Drawing for the job (mm, zero at the part's lowest x, y, z). Round coordinates to 2 decimals unless told otherwise and drop trailing zeros. Write each loop counter-clockwise with the first axis right and the second up, starting at its lowest first coordinate (ties: lowest second). Pieces come first, ordered by that corner, then holes. Notation, with made-up numbers: (4.25, -35) - (46.25, -35) arc R26 ccw to (46.25, -15) - close; hole circle Ø9 at (26, 72.25). An arc over 180 degrees is marked (long way). Answer in a Markdown table with one row per item.
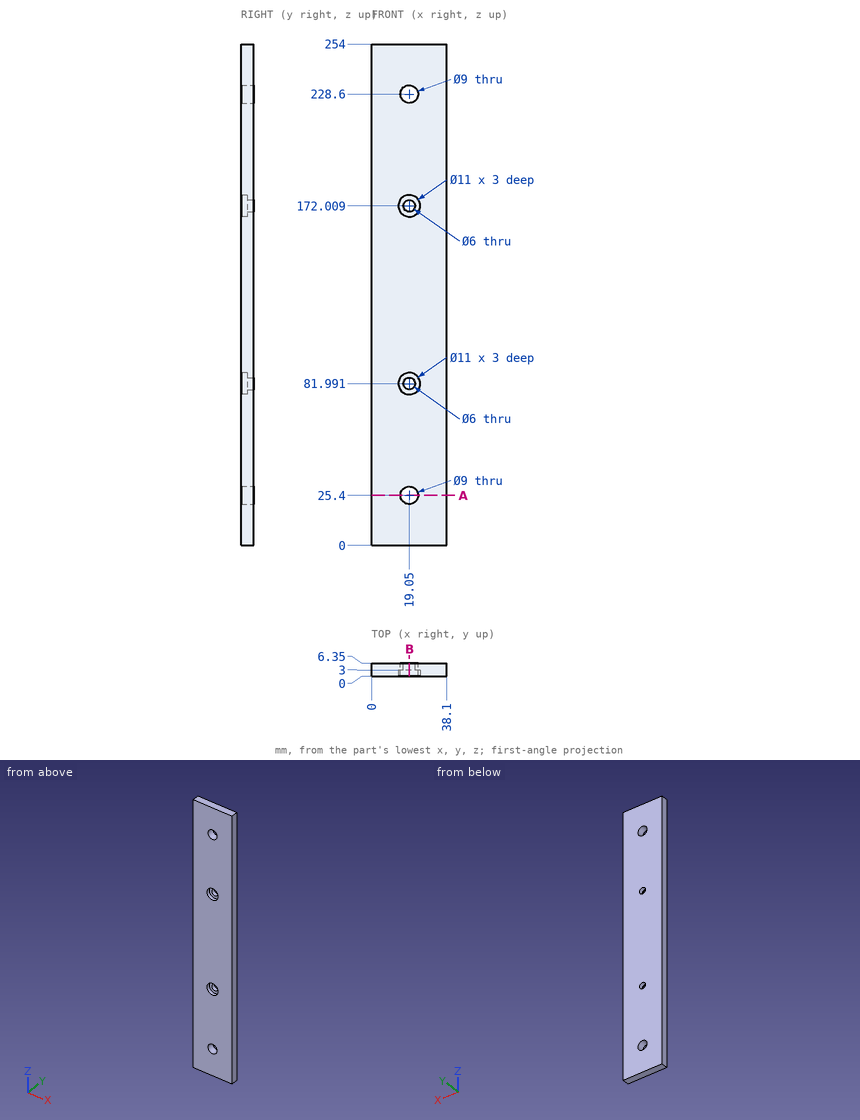
Q1. Saw through at B-B on x = 19.05. List the corners of the cut face in (y, z), then the cut area to 3 significant figures.
Computed:
| item | result |
|---|---|
| outline | (0, 0) - (6.35, 0) - (6.35, 20.9) - (0, 20.9) - close; (0, 29.9) - (6.35, 29.9) - (6.35, 78.99) - (3, 78.99) - (3, 76.49) - (0, 76.49) - close; (0, 87.49) - (3, 87.49) - (3, 84.99) - (6.35, 84.99) - (6.35, 169.01) - (3, 169.01) - (3, 166.51) - (0, 166.51) - close; (0, 177.51) - (3, 177.51) - (3, 175.01) - (6.35, 175.01) - (6.35, 224.1) - (0, 224.1) - close; (0, 233.1) - (6.35, 233.1) - (6.35, 254) - (0, 254) - close |
| area | 1,390 mm2 |
Q2. Drill centre lines: line 1 (Z direction, x = 19.05, y = 1.65); line 2 (Z direction, x = 19.05, y = 5.3); line 3 (X direction, y = 1.75, z = 224.5) (1 decimal). Where is each one in solid material? Low to high.
Computed:
| item | result |
|---|---|
| line 1 | z = 0 to 20.9, 29.9 to 76.49, 87.49 to 166.51, 177.51 to 224.1, 233.1 to 254 |
| line 2 | z = 0 to 20.9, 29.9 to 78.99, 84.99 to 169.01, 175.01 to 224.1, 233.1 to 254 |
| line 3 | x = 0 to 17.2, 20.9 to 38.1 |
Q3. Flat gauge pins, fed straight in: pin 1 (8 mm diameter, centred on x = 19.05, z = 228.6, fed in from +Y); pin 2 (3.5 mm diameter, centred on x = 20, z = 169.5, fed in from -Y). Where does each tip first touch, or does it go through?
Computed:
| item | result |
|---|---|
| pin 1 | passes through |
| pin 2 | stops at y = 3 |
Q4. Saw through at A-A on z = 25.4. List the corners of the cut face in (x, y).
Computed:
| item | result |
|---|---|
| outline | (0, 0) - (14.55, 0) - (14.55, 6.35) - (0, 6.35) - close; (23.55, 0) - (38.1, 0) - (38.1, 6.35) - (23.55, 6.35) - close |
